Autodesk Inventor part; units mm, degrees
ref_plane "YZ Plane" through (0, 0, 0) normal (1, 0, 0) x (0, 1, 0)
ref_plane "XZ Plane" through (0, 0, 0) normal (0, 1, 0) x (-1, 0, 0)
ref_plane "XY Plane" through (0, 0, 0) normal (0, 0, 1) x (1, 0, 0)
sketch "Sketch1" plane through (0, 0, 0) normal (0, 0, 1) x (1, 0, 0)
  circle A0 centre (57.407, 53.064) radius 2.5
  circle A1 centre (57.407, 53.064) radius 10
  circle A2 centre (13.407, 27.6606) radius 2.5
  circle A3 centre (13.407, 27.6606) radius 10
  circle A4 centre (57.407, 2.2572) radius 2.5
  circle A5 centre (57.407, 2.2572) radius 10
  line L0 (25.407, -164.9104) -> (25.407, 85.0896) construction
  arc A6 (64.907, 53.064) -> (53.9811, 59.7359) centre (57.407, 53.064) ccw
  arc A7 (58.5116, -5.161) -> (64.907, 2.2572) centre (57.407, 2.2572) ccw
  line L1 (10.407, 27.6606) -> (16.407, 27.6606) construction
  line L2 (10.407, 25.0106) -> (16.407, 25.0106)
  line L3 (16.407, 30.3106) -> (10.407, 30.3106)
  arc A8 (10.407, 30.3106) -> (10.407, 25.0106) centre (10.407, 27.6606) ccw
  arc A9 (16.407, 25.0106) -> (16.407, 30.3106) centre (16.407, 27.6606) ccw
  circle A10 centre (10.407, 2.8412) radius 10
  arc A11 (-3.8238, 7.5832) -> (12.6162, -11.9952) centre (10.407, 2.8412) ccw
  line L4 (12.6162, -11.9952) -> (58.5116, -5.161)
  line L5 (53.9811, 59.7359) -> (8.8392, 36.5564)
  line L6 (64.907, 2.2572) -> (64.907, 53.064)
  line L7 (3.9198, 30.8219) -> (-3.8238, 7.5832)
  line L8 (-3.8238, 7.5832) -> (-11.5466, -15.5932) construction
  line L9 (12.6162, -11.9952) -> (-11.5466, -15.5932) construction
  line L10 (-11.5466, -15.5932) -> (31.917, 20.9033) construction
  point P0 (18.407, 14.782)
  point P1 (23.5514, 8.6555)
  dimension "d52" = 15
  dimension "d53" = 15
  dimension "d54" = 3
  dimension "d55" = 5.3
  dimension "d56" = 20
  dimension "d57" = 30
  dimension "d58" = 4
  dimension "d59" = 8
extrude "Extrusion1" add sketch "Sketch1" along normal blind 4 contours A0 | L5 A6 L6 A1 | A1 L6 A5 L4 A11 L7 A3 L5 | A3 | L6 A7 L4 A5 | A4 picked at (52.4239, 56.8921) picked at (55.6672, -3.7922)
sketch "Sketch2" plane through (0, 0, 4) normal (0, 0, 1) x (1, 0, 0)
  circle A0 centre (13.407, 27.6606) radius 2.5
  circle A1 centre (57.407, 2.2572) radius 2.5
  circle A2 centre (57.407, 53.064) radius 2.5
  line L0 (10.407, 27.6606) -> (16.407, 27.6606) construction
  line L1 (10.407, 24.9106) -> (16.407, 24.9106)
  line L2 (16.407, 30.4106) -> (10.407, 30.4106)
  arc A3 (10.407, 30.4106) -> (10.407, 24.9106) centre (10.407, 27.6606) ccw
  arc A4 (16.407, 24.9106) -> (16.407, 30.4106) centre (16.407, 27.6606) ccw
  point P0 (0, 0)
  dimension "d25" = 3
  dimension "d26" = 5.5
hole "Hole2" at (57.407, 53.064, 4) at (57.407, 2.2572, 4) direction (0, 0, -1) diameter 5.5 end through all
hole "Hole4" at (18.407, 14.782, 0) at (23.5514, 8.6555, 0) direction (0, 0, 1) diameter 3 end through all
sketch "Sketch6" plane through (0, 0, 0) normal (0, 0, -1) x (-1, 0, 0)
  circle A0 centre (-49.2903, 15.4803) radius 1.7
  circle A1 centre (-30.2236, 38.1868) radius 1.7
  point P0 (0, 0)
hole "Hole6" at (49.2903, 15.4803, 0) at (30.2236, 38.1868, 0) direction (0, 0, 1) diameter 3.4 end through all countersink diameter 6.6 countersink angle 90
sketch "Sketch7" plane through (0, 0, 4) normal (0, 0, 1) x (1, 0, 0)
  point P0 (0, 0)
  point P1 (49.6217, 42.3118)
  point P2 (59.6217, 42.3118)
hole "Hole7" at (59.6217, 42.3118, 4) at (49.6217, 42.3118, 4) direction (0, 0, -1) diameter 3.4 end through all countersink diameter 6.6 countersink angle 90
properties part number "plate_3"
Geometry: final body of the model. Coordinates: model frame, mm. A direction names the side the tool comes from. Coordinates: 2 decimals unless noted, no trailing zeros. Loops run counter-clockwise (first coordinate to the right, second up) from the corner with the lowest first, then second, coordinate; pieces in that order, holes last. Notation, with made-up numbers: M -38.5,-39 L 3.5,-39 A16 cw 3.5,-34 Z; hole C 53,34 d4. An arc over 180 degrees is marked long. One line per item, written item: value. Start each with the question number.
1) Pin query (flat end, axial travel): P1, Ø1.2, axis at x = 12, z = 3, coming from the +Y side; P2, Ø5.5, axis at x = 30.22, y = 38.19, coming from the -Z side; P3, Ø3.5, axis at x = 57.407, y = 53.064, coming from the -Z side; P4, Ø1, axis at x = 16, z = 3.5, coming from the -Y side. Return the tip coordinate at first contact, or that it passes through.
2) Material intervals for L1, parallel to X at y = 1, z = 1.1; L2, parallel to Y at x = 59, z = 3.35; L3, parallel to X at y = 8.5, z = 3.85, sorted ascending. Write a range as from..to.
3) Draft query along X for faces 3 (the cylindrical face through (55.55, 55.09, 1.97)), 4 (the flat face through (35.243, -8.626, 1.972)), 5 (the cylindrical face through (61.224, 59.52, 1.972)). Return one class per face: released by +X, released by -X, zero draft, split by the parting line, or undercut.
4) Cut plane A-A (z = 0.8). Count the separate pieces of the cut face and the enclosed holes in it, then the cut area to 3 significant figures.
5) Cut plane C-C (x = 39.5). Return loops of the section in (y, z).
6) Cut plane B-B (y = 34). Return loops of the section in (x, z), then the cut area to 3 significant figures.
7) Reachability of faces 1 (the flat face through (37, 25, 0)), 2 (the cylindrical face through (19.056, 27.719, 1.972)) from +Z, -Z, +X, -X, +Y, -Y: full face, straight path, thin tool, end or side. Return the list, or none.
Evaluation:
1. P1: y = 38.49
1. P2: z = 0.55
1. P3: through
1. P4: y = -11.57
2. L1: -4.48..0.58, 20.24..54.96, 59.85..64.8
2. L2: -5.07..0.02, 4.5..39.74, 44.89..50.82, 55.31..60.39
2. L3: -3.52..2.16, 18.65..22.06, 25.04..64.91
3. face 3: undercut
3. face 4: released by +X
3. face 5: split by the parting line
4. separate pieces: 1
4. enclosed holes: 10
4. area: 3,230 mm^2
5. outline: M -7.99,0 L 52.3,0 L 52.3,4 L -7.99,4 Z
6. outline: M 5.67,0 L 64.91,0 L 64.91,4 L 5.67,4 Z
6. area: 237 mm^2
7. face 1: -Z, +X, -X, +Y, -Y
7. face 2: +Z, -Z
